Autodesk Inventor part; units mm, degrees
ref_plane "Work Plane1" through (0, -5, 0) normal (0, -1, 0) x (1, 0, 0)
ref_plane "Work Plane3" through (0, -35, 0) normal (0, -1, 0) x (1, 0, 0)
ref_plane "Work Plane4" through (0, -35, 0) normal (0, -1, 0) x (1, 0, 0)
sketch "Sketch1" plane through (0, 0, 0) normal (0, 1, 0) x (-1, 0, 0)
  line L0 (30, 0) -> (-30, 0) construction
  arc A0 (-30, 32.5) -> (-30, -32.5) centre (-30, 0) ccw
  circle A1 centre (-30, 0) radius 32.5 construction
  circle A2 centre (-30, 0) radius 30 construction
  circle A3 centre (-30, -6.25) radius 2
  circle A4 centre (-30, 6.25) radius 2
  arc A5 (-15.4703, 26.2467) -> (-59.998, -0.3452) centre (-30, 0) ccw
  arc A6 (-3.6144, 14.2758) -> (-15.4703, 26.2467) centre (-30, 0) ccw
  arc A7 (-2.1644, 16.7758) -> (-30, 32.5) centre (-30, 0) ccw
  line L1 (-30, -6.25) -> (-30, 6.25) construction
  line L2 (-30, 0) -> (-36.25, 0) construction
  line L3 (-30, 0) -> (-23.75, 0) construction
  line L4 (-30, 0) -> (-23.75, 0) construction
  circle A8 centre (-23.75, 0) radius 2
  circle A9 centre (-36.25, 0) radius 2
  line L5 (-30, 0) -> (-30, -6.25) construction
  line L6 (-3.6144, 14.2758) -> (-3.6144, -14.2758) construction
  line L7 (-2.1644, 16.7758) -> (-2.1644, -16.7758) construction
  line L8 (-30, 32.5) -> (52.5439, 32.5) construction
  line L9 (-2.1644, 16.7758) -> (17.8356, 16.7758) construction
  line L10 (17.8356, 16.7758) -> (17.8356, -16.7758) construction
  line L11 (17.8356, -16.7758) -> (-2.1644, -16.7758) construction
  line L12 (-3.6144, -14.2758) -> (19.2856, -14.2758) construction
  line L13 (19.2856, -14.2758) -> (19.2856, 14.2758) construction
  line L14 (-3.6144, 14.2758) -> (19.2856, 14.2758) construction
  line L15 (0, 16.7758) -> (0, -16.7758) construction
  line L16 (2.5, 0) -> (2.5, 16.7758) construction
  line L17 (2.5, 0) -> (2.5, -16.7758) construction
  line L18 (19.2856, 0) -> (21.4496, 0) construction
  line L19 (21.4496, 0) -> (21.4496, 16.7758) construction
  line L20 (21.4496, 16.7758) -> (17.8356, 16.7758) construction
  line L21 (19.2856, 14.2758) -> (19.2856, 16.7758) construction
  line L22 (21.4496, 0) -> (21.4496, -16.7758) construction
  line L23 (21.4496, -16.7758) -> (17.8356, -16.7758) construction
  line L24 (19.2856, -14.2758) -> (19.2856, -16.7758) construction
  line L25 (21.4496, 0) -> (51.4496, 0) construction
  circle A10 centre (51.4496, 0) radius 30 construction
  circle A11 centre (51.4496, 0) radius 32.5 construction
  line L26 (19.2856, 14.2758) -> (25.064, 14.2758) construction
  line L27 (20.3676, 16.7758) -> (23.614, 16.7758) construction
  line L28 (17.3742, -16.7758) -> (23.614, -16.7758) construction
  line L29 (17.8356, -14.2758) -> (22.2529, -14.2758) construction
  line L30 (22.2529, -14.2758) -> (25.064, -14.2758) construction
  arc A12 (81.4496, 0) -> (51.4496, 30) centre (51.4496, 0) ccw
  arc A13 (51.4496, -30) -> (81.4496, 0) centre (51.4496, 0) ccw
  line L31 (51.4496, 30) -> (51.4496, -30) construction
  arc A14 (51.4496, 30) -> (25.064, 14.2758) centre (51.4496, 0) ccw
  line L32 (25.064, 14.2758) -> (-3.6144, 14.2758)
  line L33 (23.614, 16.7758) -> (-2.1644, 16.7758)
  arc A15 (51.4496, -32.5) -> (83.9496, 0) centre (51.4496, 0) ccw
  arc A16 (83.9496, 0) -> (51.4496, 32.5) centre (51.4496, 0) ccw
  arc A17 (51.4496, 32.5) -> (23.614, 16.7758) centre (51.4496, 0) ccw
  circle A18 centre (51.4496, 0) radius 15
  line L34 (51.4496, -32.5) -> (-30, -32.5)
  line L35 (51.4496, -30) -> (-30, -30)
  arc A19 (-59.998, -0.3452) -> (-30, -30) centre (-30, 0) ccw
  point P0 (0, 0)
  point P1 (-30, 32.5)
  point P2 (-25, 0)
  point P3 (7.8356, 16.7758)
  dimension "d1" = 30
  dimension "d2" = 65
  dimension "d12" = 60
  dimension "d25" = 4
  dimension "d28" = 4
  dimension "d51" = 12.5
  dimension "d60" = 6.25
  dimension "d61" = 180
  dimension "d62" = 6.25
  dimension "d63" = 4
  dimension "d64" = 4
  dimension "d65" = 6.25
  dimension "d68" = 20
  dimension "d69" = 1.45
  dimension "d70" = 1.45
  dimension "d71" = 2.5
  dimension "d72" = 2.5
  dimension "d73" = 2.1644
  dimension "d74" = 2.164
  dimension "d75" = 30
  dimension "d76" = 60
  dimension "d77" = 65
  dimension "d78" = 60
  dimension "d79" = 30
ref_plane "Work Plane1" through (0, -5, 0) normal (0, -1, 0) x (1, 0, 0)
ref_plane "Work Plane3" through (0, -35, 0) normal (0, -1, 0) x (1, 0, 0)
sketch "Sketch3" plane through (0, -35, 0) normal (0, -1, 0) x (1, 0, 0)
  point P0 (0, 0)
extrude "Extrusion12" add sketch "Sketch1" against normal blind 2.5 contours A6 L32 A14 A12 A13 L35 A19 A5
extrude "Extrusion13" add sketch "Sketch1" against normal blind 35 contours A7 L33 A17 A16 A15 L34 A0
ref_plane "Work Plane4" through (0, -35, 0) normal (0, -1, 0) x (1, 0, 0)
sketch "Sketch5" plane through (0, -35, 0) normal (0, -1, 0) x (1, 0, 0)
  line L0 (-25.064, 14.2758) -> (3.6144, 14.2758) construction
  line L1 (30, -30) -> (-51.4496, -30) construction
  line L2 (3.6144, 14.2758) -> (-51.4496, -30) construction
  line L3 (-25.064, 14.2758) -> (30, -30) construction
  line L4 (-10.7248, 14.2758) -> (-10.7248, -30) construction
  line L5 (30, -30) -> (30, 30) construction
  arc A0 (30, -30) -> (3.6144, 14.2758) centre (30, 0) ccw construction
  arc A1 (-25.064, 14.2758) -> (-51.4496, -30) centre (-51.4496, 0) ccw construction
  line L6 (-51.4496, -30) -> (-51.4496, 30) construction
  arc A2 (-23.614, 16.7758) -> (-51.4496, -32.5) centre (-51.4496, 0) ccw construction
  arc A3 (30, -32.5) -> (2.1644, 16.7758) centre (30, 0) ccw construction
  line L7 (62.5, 0) -> (60, 0) construction
  line L8 (30, -30) -> (30, -32.5) construction
  line L9 (-51.4496, -30) -> (-51.4496, -32.5) construction
  line L10 (-51.4496, 30) -> (-51.4496, 32.5) construction
  line L11 (30, 30) -> (30, 32.5) construction
  line L12 (-10.7248, -30) -> (-10.7248, -32.5) construction
  line L13 (30, -32.5) -> (-51.4496, -32.5) construction
  line L14 (-10.7248, 14.2758) -> (-10.7248, 16.7758) construction
  circle A4 centre (-10.7248, 15.5258) radius 0.5
  circle A5 centre (30, 31.25) radius 0.5
  circle A6 centre (61.25, 0) radius 0.5
  circle A7 centre (30, -31.25) radius 0.5
  circle A8 centre (-51.4496, -31.25) radius 0.5
  circle A9 centre (-51.4496, 31.25) radius 0.5
  line L15 (30, 31.25) -> (-51.4496, 31.25) construction
  line L16 (59.4615, 0) -> (-81.4496, 0) construction
  line L17 (-81.4496, 0) -> (-83.9496, 0) construction
  circle A10 centre (-82.6996, 0) radius 0.5
  point P0 (0, 0)
  dimension "d100" = 1
  dimension "d101" = 1
  dimension "d102" = 1
  dimension "d103" = 1
  dimension "d104" = 1
  dimension "d105" = 1
  dimension "d106" = 81.4496
  dimension "d108" = 140.9111
  dimension "d109" = 1
extrude "Extrusion14" cut sketch "Sketch5" against normal blind 15
properties part number "con_v6_d1_3DPrint"
Work out the finished part from the listing and answer in its coordinate system (mm). A direction names the side the tool comes from. Round coordinates to 2 decimals unless told otherwise and drop trailing zeros. Write each loop counter-clockwise with the first axis right and the second up, starting at its lowest first coordinate (ties: lowest second). Pieces come first, ordered by that corner, then holes. Notation, with made-up numbers: (75, 45.25) - (124, 45.25) arc R20 ccw to (124, 77.25) - close; hole circle Ø7 at (38, -23). An arc over 180 degrees is marked (long way). Return JSON: item names as keys, results as strings. Group by question number.
Q1. For faces 4 (the cylindrical face through (38.248, -1.232, 0.088)), 5 (the cylindrical face through (-35.67, -17.26, 28.41)), 6 (the flat face through (-10, -2.5, 0)), determine the directions among +Z, -Z, +X, -X, +Y, -Y from which every point of the face is accessible in a straight line to the end or side of a thin tool.
Q2. The part is cut by section B-B on x = -45.5. Write down the section's boundary in (y, z), then the cut area to 3 significant figures.
Q3. Find the intervals of material crossed by L1, parallel to Z at x = -52, y = -8.5; L2, parallel to Z at x = -1.5, y = -19; L3, parallel to X at y = -11, z = 16, in increasing order.
Q4. The mould has two halves that part along X. Classify faces 1 (the cylindrical face through (45, -18.52, 25.98)), 2 (the cylindrical face through (62.492, -17.255, 0.715)), 3 (the flat face through (-10, -35, 15)): released by +X, released by -X, zero draft, split by the parting line, or undercut.
Q5. The part is cut by section D-D on z = -6.25. Write down the section's boundary in (x, y), then the cut area to 3 significant figures.
Q6. The part is cut by section C-C on y = -18. Write down the section's boundary in (x, z), then the cut area to 3 significant figures.
Q7. Each of these flat-tipped pins is pushed along its axis until it touches: pin 1 Ø1 at (x, z) = (33, 3) entering from -Y; pin 2 Ø0.8 at (x, z) = (61, 0) entering from -Y; pin 3 Ø16 at (x, y) = (-3.5, -12) entering from +Z; pin 4 Ø4 at (x, y) = (20, -14) entering from +Z. Where does it stop, or does it pass through?
Q8. The part is cut by section A-A on z = 24.5. Write down the section's boundary in (x, y).
Solved:
{
 "1": {"face 4": "+Y, -Y", "face 5": "+Z, +Y, -Y", "face 6": "-Y"},
 "2": {"outline": "(-35, -32.5) - (0, -32.5) - (0, -13.77) - (-2.5, -13.77) - (-2.5, -30) - (-35, -30) - close; (-35, 29.4) - (-2.5, 29.4) - (-2.5, 13.77) - (0, 13.77) - (0, 31.95) - (-35, 31.95) - close", "area": "256 mm²"},
 "3": {"L1": "-32.5 to -29.99, 29.99 to 32.5", "L2": "-32.5 to -30, 14.28 to 16.78", "L3": "-79.74 to -76.83, -26.07 to 4.62, 55.38 to 58.29"},
 "4": {"face 1": "undercut", "face 2": "released by +X", "face 3": "zero draft"},
 "5": {"outline": "(-83.34, -35) - (-80.79, -35) - (-80.79, -2.5) - (-65.09, -2.5) - (-65.09, 0) - (-83.34, 0) - close; (-37.81, -2.5) - (28, -2.5) - (28, 0) - (-37.81, 0) - close; (32, -2.5) - (59.34, -2.5) - (59.34, -35) - (61.89, -35) - (61.89, 0) - (32, 0) - close", "area": "451 mm²"},
 "6": {"outline": "(-51.45, -32.5) - (30, -32.5) arc R32.5 ccw to (30, 32.5) arc R32.5 ccw to (2.16, 16.78) - (-23.61, 16.78) arc R32.5 ccw to (-51.45, 32.5) arc R32.5 ccw to start; hole (-51.45, -30) - (30, -30) arc R30 ccw to (60, -0.35) arc R30 ccw to (15.47, 26.25) arc R30 ccw to (3.61, 14.28) - (-25.06, 14.28) arc R30 ccw to (-51.45, 30) arc R30 ccw to start", "area": "927 mm²"},
 "7": {"pin 1": "y = -2.5", "pin 2": "y = -35", "pin 3": "z = 20.15", "pin 4": "z = 31.5"},
 "8": {"outline": "(-72.8, -35) - (-68.76, -35) - (-68.76, -2.5) - (-34.14, -2.5) - (-34.14, -35) - (-30.1, -35) - (-30.1, 0) - (-72.8, 0) - close; (8.65, -35) - (12.69, -35) - (12.69, -2.5) - (47.31, -2.5) - (47.31, -35) - (51.35, -35) - (51.35, 0) - (8.65, 0) - close"}
}
